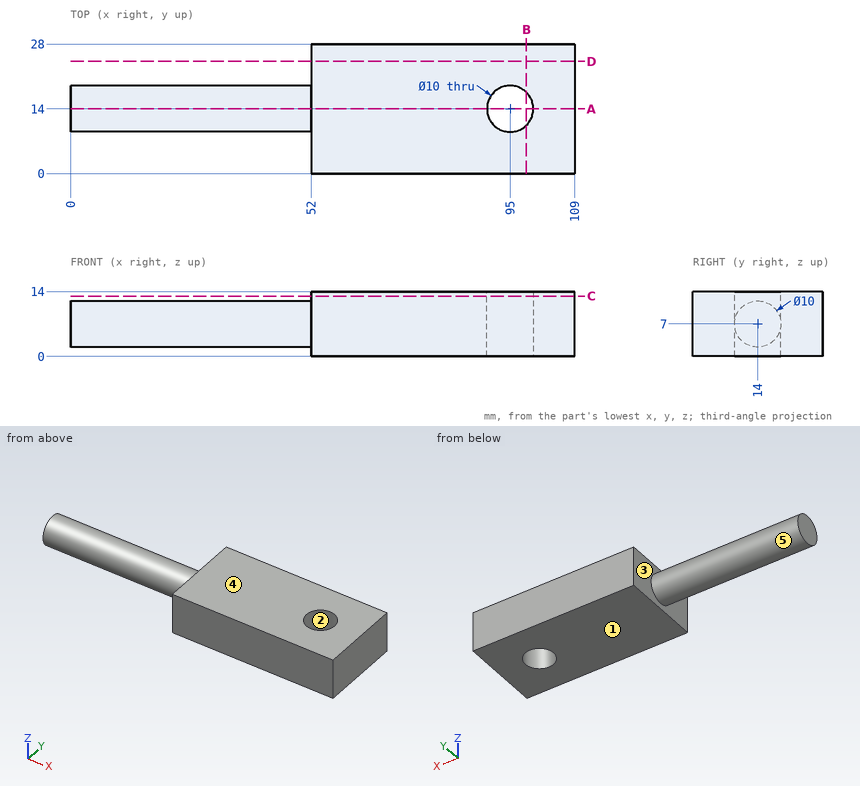
Could you check a few things on this drawing? It's one solid part, dimensions in mm from its lowest x, y, z. A direction names the side the tool comes from. Give positions to 0.01 mm unless a question says otherwise; leave off trailing zeros. Order: outer loops, then holes, each group sorted by start corner. A loop starts at its lowest first (then second) coordinate and runs counter-clockwise, first axis right, second up. Notation, with made-up numbers: (41, 80.5) -> (84, 80.5) arc R27 cw to (84, 114.5) -> close; hole circle Ø9 at (68.5, 15.5). An arc over 180 degrees is marked (long way). Answer in a Markdown table with one row per item. Add a question column.
Item 1: Please list where these lines run through material, in increasing order: probe 1 along Y at (x, z) = (95, 5.5); probe 2 along X at (y, z) = (27, 12); probe 3 along X at (y, z) = (9.75, 1.25).
Item 2: Imagine slicing it at C-C (z = 13). List the corners of the cut face in (x, y) for me.
Item 3: Imagine slicing it at D-D (y = 24.25). List the corners of the cut face in (x, z) for me.
Item 4: I'm going to push flat-ended pins straight in: P1, Ø2, axis at y = 22, z = 9, coming from the -X side; P2, Ø9, axis at x = 95, y = 14, coming from the -Z side; P3, Ø1.5, axis at x = 38, y = 19, coming from the -Z side; P4, Ø5, axis at x = 35.5, z = 6, coming from the +Y side. Where does each tip first touch, or does it pass through?
Item 5: We'd pull the mould along X, two halves only. Please class the marked faces 1, 2 and 3: pulls with the +X half, pulls with the -X half, needs draft (parallel to the pull), parting line crosses it, or undercut.
Item 6: Imagine slicing it at A-A (y = 14). List the corners of the cut face in (x, z) for me, and give its area (3 significant figures).
Item 7: Imagine slicing it at B-B (x = 98.5). List the corners of the cut face in (y, z) for me, and give its area (3 significant figures).
Item 8: For the marked faces 4 and 5, which set-ups out of +Z, -Z, +X, -X, +Y, -Y let a thin tool reach every point of the face, with its end or its side?
Result:
| question | item | result |
|---|---|---|
| 1 | probe 1 | 0 to 9, 19 to 28 |
| 1 | probe 2 | 52 to 109 |
| 1 | probe 3 | 52 to 92.37, 97.63 to 109 |
| 2 | outline | (52, 0) -> (109, 0) -> (109, 28) -> (52, 28) -> close; hole circle Ø10 at (95, 14) |
| 3 | outline | (52, 0) -> (109, 0) -> (109, 14) -> (52, 14) -> close |
| 4 | P1 | x = 52 |
| 4 | P2 | through |
| 4 | P3 | z = 4.37 |
| 4 | P4 | y = 19 |
| 5 | face 1 | needs draft |
| 5 | face 2 | undercut |
| 5 | face 3 | pulls with the -X half |
| 6 | outline | (0, 2) -> (52, 2) -> (52, 0) -> (90, 0) -> (90, 14) -> (52, 14) -> (52, 12) -> (0, 12) -> close; (100, 0) -> (109, 0) -> (109, 14) -> (100, 14) -> close |
| 6 | area | 1,180 mm2 |
| 7 | outline | (0, 0) -> (10.43, 0) -> (10.43, 14) -> (0, 14) -> close; (17.57, 0) -> (28, 0) -> (28, 14) -> (17.57, 14) -> close |
| 7 | area | 292 mm2 |
| 8 | face 4 | +Z, +X, -X, +Y, -Y |
| 8 | face 5 | -X |
